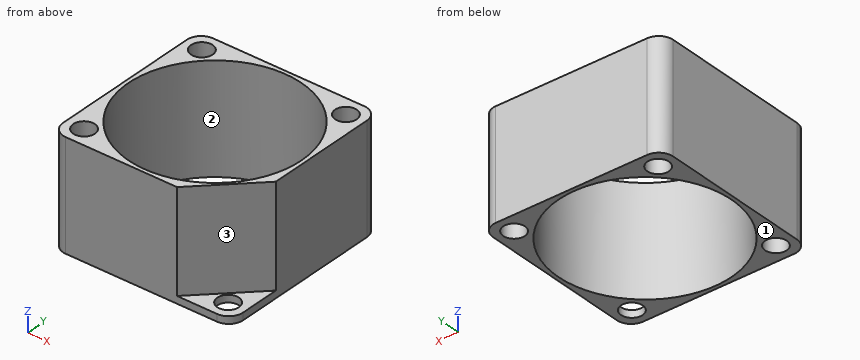
Autodesk Inventor part; units mm, degrees
ref_plane "YZ Plane" through (0, 0, 0) normal (1, 0, 0) x (0, 1, 0)
ref_plane "XZ Plane" through (0, 0, 0) normal (0, 1, 0) x (-1, 0, 0)
ref_plane "XY Plane" through (0, 0, 0) normal (0, 0, 1) x (1, 0, 0)
sketch "Sketch1" plane through (0, 0, 0) normal (0, 0, 1) x (1, 0, 0)
  line L0 (-12.5, 12.5) -> (12.5, 12.5)
  line L1 (12.5, 12.5) -> (12.5, -12.5)
  line L2 (12.5, -12.5) -> (-12.5, -12.5)
  line L3 (-12.5, -12.5) -> (-12.5, 12.5)
  line L4 (-12.5, 12.5) -> (12.5, -12.5) construction
  line L5 (12.5, 12.5) -> (-12.5, -12.5) construction
  point P0 (0, 0)
  dimension "d0" = 25
  dimension "d1" = 25
extrude "Extrusion1" add sketch "Sketch1" along normal blind 15
sketch "Sketch2" plane through (0, 0, 15) normal (0, 0, 1) x (1, 0, 0)
  line L0 (-10, -10) -> (10, -10)
  line L1 (10, -10) -> (10, 10)
  line L2 (10, 10) -> (-10, 10)
  line L3 (-10, 10) -> (-10, -10)
  line L4 (-10, -10) -> (10, 10) construction
  line L5 (10, -10) -> (-10, 10) construction
  point P0 (0, 0)
  dimension "d4" = 20
  dimension "d5" = 20
hole "Hole1" at (-10, 10, 15) at (10, 10, 15) at (10, -10, 15) at (-10, -10, 15) direction (0, 0, -1) diameter 3 end through all
fillet "Fillet1" radius 2 4 edges at (-12.5, 12.5, 7.5) (-12.5, -12.5, 7.5) (12.5, -12.5, 7.5) (12.5, 12.5, 7.5)
sketch "Sketch3" plane through (0, 0, 15) normal (0, 0, 1) x (1, 0, 0)
  circle A0 centre (0, 0) radius 12
  dimension "d14" = 24
extrude "Extrusion2" cut sketch "Sketch3" against normal through all
sketch "Sketch4" plane through (0, 0, 15) normal (0, 0, 1) x (1, 0, 0)
  line L0 (-10.5, -12.5) -> (10.5, -12.5)
  line L1 (4.9555, -12.5) -> (12.5, -4.9555)
  line L2 (12.5, -10.5) -> (12.5, 10.5)
  arc A0 (10.5, -12.5) -> (12.5, -10.5) centre (10.5, -10.5) ccw
  point P0 (0, 0)
  dimension "d17" = 45
extrude "Extrusion3" cut sketch "Sketch4" against normal blind 14
properties part number "MF25150V1-1000U-A99" material "ABS Plastic"
Model file for the job. Use its own axes, mm. Face numbers are marked on the shaded views. Give positions to 0.01 mm unless a question says otherwise; leave off trailing zeros. Order: outer loops, then holes, each group sorted by start corner. A loop starts at its lowest first (then second) coordinate and runs counter-clockwise, first axis right, second up. Notation, with made-up numbers: M 49.5,-2.5 L 90.5,-2.5 A21 cw 90.5,11.5 Z; hole C -6,50 d1. An arc over 180 degrees is marked long. Put each result on its own line as item: value. Start each with the question number.
(1) Pull direction Y, two halves, no side cores. Call the marked faces 1, 2 and 3: released by +Y, released by -Y, zero draft, split by the parting line, or undercut.
(2) Band-saw the part on C-C on z = 1.5. Give the cut face in (x, y), then the cut area to 3 significant figures.
(3) Drill centre lines: L1, parallel to Y at x = 0, z = 7; L2, parallel to X at y = -9, z = 11; L3, parallel to X at y = -10, z = 6. Where is each one in solid material? Low to high. Write a range as [from, to].
(4) Band-saw the part on D-D on y = -10. Give the cut face in (x, z).
(5) Band-saw the part on B-B on x = 10. Give the cut face in (y, z).
(6) Pin check, flat tip, straight feed: pin 1 Ø12 at (x, y) = (0, -7) entering from +Z. Stop position of the tip, or through.
(7) Band-saw the part on A-A on y = 0. Give the cut face in (x, z), then the cut area to 3 significant figures.
Results below:
1. face 1: zero draft
1. face 2: undercut
1. face 3: released by -Y
2. outline: M -12.5,-10.5 A2 ccw -10.5,-12.5 L 4.96,-12.5 L 12.5,-4.96 L 12.5,10.5 A2 ccw 10.5,12.5 L -10.5,12.5 A2 ccw -12.5,10.5 Z; hole C 0,0 d24; hole C -10,-10 d3; hole C -10,10 d3; hole C 10,10 d3
2. area: 120 mm2
3. L1: y = [-12.5, -12], [12, 12.5]
3. L2: x = [-12.5, -11.12], [-8.88, -7.94], [7.94, 8.46]
3. L3: x = [-12.5, -11.5], [-8.5, -6.63], [6.63, 7.46]
4. outline: M -12.5,0 L -11.5,0 L -11.5,15 L -12.5,15 Z; M -8.5,0 L -6.63,0 L -6.63,15 L -8.5,15 Z; M 6.63,0 L 8.5,0 L 8.5,1 L 7.46,1 L 7.46,15 L 6.63,15 Z; M 11.5,0 L 12.5,0 L 12.5,1 L 11.5,1 Z
5. outline: M -12.5,0 L -11.5,0 L -11.5,1 L -12.5,1 Z; M -8.5,0 L -6.63,0 L -6.63,15 L -7.46,15 L -7.46,1 L -8.5,1 Z; M 6.63,0 L 8.5,0 L 8.5,15 L 6.63,15 Z; M 11.5,0 L 12.5,0 L 12.5,15 L 11.5,15 Z
6. pin 1: stops at z = 15
7. outline: M -12.5,0 L -12,0 L -12,15 L -12.5,15 Z; M 12,0 L 12.5,0 L 12.5,15 L 12,15 Z
7. area: 15.0 mm2
